```python
from build123d import *

# Parameters (mm, degrees)
F2_R     = 6.5
F2_R_2   = 4.5
F3_DEPTH = 9
F4_DEPTH = 20.001


with BuildPart() as f1:
    # F0 (on Front) → F1 (revolve)
    with BuildSketch(Plane.XZ):
        Polygon((0, 50), (0, 6), (20, 6), (20, 10), (12, 10), (12, 50), align=None)
    revolve(axis=Axis((26.5880525112, 0, 0), (1, 0, 0)))

    # F2 (on face) → F3 (cut)
    with BuildSketch(Plane(origin=(0, 0, 0), x_dir=(0, -1, 0), z_dir=(-1, 0, 0))):
        with Locations((0, 35)):
            Circle(F2_R)
        with Locations((0, 35)):
            Circle(F2_R_2, mode=Mode.SUBTRACT)
        with Locations((-35, 0)):
            Circle(F2_R)
        with Locations((-35, 0)):
            Circle(F2_R_2, mode=Mode.SUBTRACT)
        with Locations((0, -35)):
            Circle(F2_R)
        with Locations((0, -35)):
            Circle(F2_R_2, mode=Mode.SUBTRACT)
        with Locations((35, 0)):
            Circle(F2_R)
        with Locations((35, 0)):
            Circle(F2_R_2, mode=Mode.SUBTRACT)
    extrude(amount=-F3_DEPTH, mode=Mode.SUBTRACT)

    # F4 (cut, through all): faces of the model
    f4_faces = [f1.faces().sort_by_distance(p)[0] for p in [
        (0, 0, 35),
        (0, 35, 0),
        (0, 0, -35),
        (0, -35, 0),
    ]]
    extrude(f4_faces, amount=-F4_DEPTH, mode=Mode.SUBTRACT)


solid = f1.part
```
Input: part model. Units: mm. Frame: model coordinates. A direction names the side the tool comes from. Give positions to 0.01 mm unless a question says otherwise; leave off trailing zeros. Order: outer loops, then holes, each group sorted by start corner. A loop starts at its lowest first (then second) coordinate and runs counter-clockwise, first axis right, second up. Notation, with made-up numbers: M 82.5,53 L 108.5,53 A20 ccw 108.5,76 Z; hole C 49.25,53 d9. An arc over 180 degrees is marked long. One line per question, with ' | ' between items. Start each with the question number.
1. Section query C-C (y = -38). Return the cut outline in (x, z).
2. Access query for faces 4 (the face through (4.437, 0.846, 41.445)), 5 (the face through (10.479, 30.708, 1.352)). Directions: +Z, -Z, +X, -X, +Y, -Y. A direction counts if a zero-diameter tool reaches every point of the face in a straight line with its end or side. Return the directions, or none.
3. Section query D-D (x = 4.25). Return the cut outline in (y, z), and give its area (3 significant figures).
4. Section query A-A (y = 0). Return the cut outline in (x, z).
5. Pull-direction query (Z, two-part tool) for faces 1 (the face through (10.48, 0.98, 30.61)), 2 (the face through (15.94, 9.76, -2.17)), 3 (the face through (20, 0, -7)); classes: released by +Z, released by -Z, zero draft, split by the parting line, or undercut.
6. First-contact query: pin 1 Ø11.5 at (y, z) = (0, 35) entering from +X; pin 2 Ø12 at (x, z) = (8, 35) entering from +Y; pin 3 Ø11.5 at (y, z) = (0, 35) entering from -X; pin 4 Ø7 at (y, z) = (35, 0) entering from +X. Flat tips, straight axial feed; report the tip coordinate or a pass-through.
7. Material intervals for probe 1 along X at (y, z) = (21, -39.5); probe 2 along X at (y, z) = (-29.5, -2.5); probe 3 along Z at (x, y) = (8.5, 31), sorted ascending. Write a range as [from, to].
Here are the results:
1) outline: M 0,-32.5 L 12,-32.5 L 12,-3.35 L 9,-3.35 L 9,-5.77 L 0,-5.77 Z; M 0,5.77 L 9,5.77 L 9,3.35 L 12,3.35 L 12,32.5 L 0,32.5 Z
2) face 4: -X | face 5: +X, -X
3) outline: C 0,0 d100; hole C -35,0 d13; hole C 0,-35 d13; hole C 0,35 d13; hole C 0,0 d12; hole C 35,0 d13 | area: 7,210 mm²
4) outline: M 0,-50 L 12,-50 L 12,-39.5 L 9,-39.5 L 9,-41.5 L 0,-41.5 Z; M 0,-28.5 L 9,-28.5 L 9,-30.5 L 12,-30.5 L 12,-10 L 20,-10 L 20,-6 L 0,-6 Z; M 0,6 L 20,6 L 20,10 L 12,10 L 12,30.5 L 9,30.5 L 9,28.5 L 0,28.5 Z; M 0,41.5 L 9,41.5 L 9,39.5 L 12,39.5 L 12,50 L 0,50 Z
5) face 1: undercut | face 2: split by the parting line | face 3: zero draft
6) pin 1: x = 12 | pin 2: y = 40.73 | pin 3: x = 9 | pin 4: through
7) probe 1: [0, 12] | probe 2: [9, 12] | probe 3: [-39.23, -5.12], [5.12, 39.23]
